Read the model definition and answer for the solid it produces. Units are mm, in the model's axes. A direction names the side the tool comes from. Coordinates: 2 decimals unless noted, no trailing zeros. Loops run counter-clockwise (first coordinate to the right, second up) from the corner with the lowest first, then second, coordinate; pieces in that order, holes last.
Q1. A straight line is drawn through the part: line 1 (Y direction, x = 104, z = 94). Find the intervals that lie inside material, in ascending order.
Q2. Section B-B (z = 82) is taken. Give the vertices of the cut face in (x, y), then the cut area to 3 significant figures.
Q3. The mould has two halves that part along X. Classify faces 1 (the face through (500, -7, 49)), 2 (the face through (-2, 152.5, 49)), 3 (the face through (-7, -500, 49)), 4 (the face through (-500, -7, 49)): pulls with the +X half, pulls with the -X half, needs draft (parallel to the pull), parting line crosses it, or undercut.
Q4. Which of the six approach directions +Z, -Z, +X, -X, +Y, -Y give full straight-line access (tool end or side, diameter ignored) to faces 5 (the face through (-2, -152.5, 49)), 6 (the face through (-227, 7, 0))?
Q5. Section A-A (x = 132) is taken. Give the vertices of the cut face in (y, z).
from build123d import *

# Parameters (mm, degrees)
F0_W     = 1000
F0_H     = 1000
F0_W_2   = 305
F0_H_2   = 305
F1_DEPTH = 100
F2_R     = 5


with BuildPart() as f1:
    # F0 (on Top) → F1 (new body)
    with BuildSketch(Plane.XY):
        Rectangle(F0_W, F0_H)
        Rectangle(F0_W_2, F0_H_2, mode=Mode.SUBTRACT)
    extrude(amount=F1_DEPTH)

    # F2
    f2_edges = [f1.edges().sort_by_distance(p)[0] for p in [
        (500, 0, 100),
        (0, 500, 100),
        (-500, 0, 100),
        (0, -500, 100),
        (0, 152.5, 100),
        (152.5, 0, 100),
        (0, -152.5, 100),
        (-152.5, 0, 100),
        (500, 0, 0),
        (0, 500, 0),
        (-500, 0, 0),
        (0, -500, 0),
        (0, 152.5, 0),
        (152.5, 0, 0),
        (0, -152.5, 0),
        (-152.5, 0, 0),
        (-152.5, 152.5, 50),
        (152.5, 152.5, 50),
        (152.5, -152.5, 50),
        (-152.5, -152.5, 50),
        (500, 500, 50),
        (-500, 500, 50),
        (-500, -500, 50),
        (500, -500, 50),
    ]]
    fillet(f2_edges, radius=F2_R)


solid = f1.part
Numbers:
1. line 1: y = -500 to -152.5, 152.5 to 500
2. outline: (-500, -495) arc R5 ccw to (-495, -500) - (495, -500) arc R5 ccw to (500, -495) - (500, 495) arc R5 ccw to (495, 500) - (-495, 500) arc R5 ccw to (-500, 495) - close; hole (-152.5, -147.5) arc R5 ccw to (-147.5, -152.5) - (147.5, -152.5) arc R5 ccw to (152.5, -147.5) - (152.5, 147.5) arc R5 ccw to (147.5, 152.5) - (-147.5, 152.5) arc R5 ccw to (-152.5, 147.5) - close
2. area: 907,000 mm2
3. face 1: pulls with the +X half
3. face 2: undercut
3. face 3: needs draft
3. face 4: pulls with the -X half
4. face 5: +Z, -Z
4. face 6: -Z, +X, -X, +Y, -Y
5. outline: (-500, 5) arc R5 ccw to (-495, 0) - (-157.5, 0) arc R5 ccw to (-152.5, 5) - (-152.5, 95) arc R5 ccw to (-157.5, 100) - (-495, 100) arc R5 ccw to (-500, 95) - close; (152.5, 5) arc R5 ccw to (157.5, 0) - (495, 0) arc R5 ccw to (500, 5) - (500, 95) arc R5 ccw to (495, 100) - (157.5, 100) arc R5 ccw to (152.5, 95) - close
